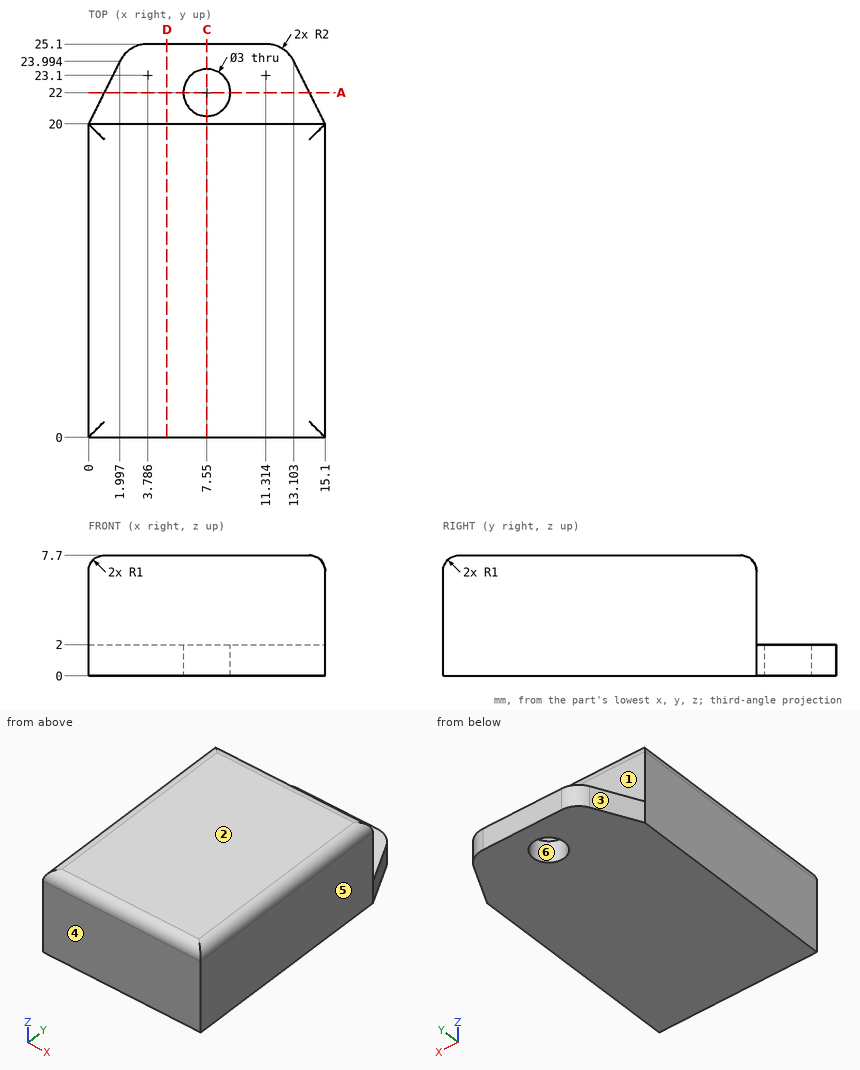
Drawing for the job (mm, zero at the part's lowest x, y, z). A direction names the side the tool comes from. Round coordinates to 2 decimals unless told otherwise and drop trailing zeros. Write each loop counter-clockwise with the first axis right and the second up, starting at its lowest first coordinate (ties: lowest second). Pieces come first, ordered by that corner, then holes. Notation, with made-up numbers: (1.5, 15) - (43.5, 15) arc R20 cw to (43.5, 26) - close; hole circle Ø11 at (-13, -30.5). An arc over 180 degrees is marked (long way). Write item = value, one per line. Start each with the question number.
Q1. Mould opens along X. For the marked faces 3, 4, 5 and 6 say: pulls with the +X half, pulls with the -X half, needs draft (parallel to the pull), parting line crosses it, or undercut.
Q2. Drop flat-ended pins along their axis: pin 1 (3 mm diameter, centred on x = 8.5, y = 5, fed in from -Z); pin 2 (2.5 mm diameter, centred on x = 6.5, y = 22, fed in from +Z). Give the stop position or say it passes through.
Q3. Band-saw the part on C-C (x = 7.55). Give the cut face in (y, z).
Q4. Band-saw the part on A-A (y = 22). Give the cut face in (x, z), then the cut area to 3 significant figures.
Q5. Which spindle directions (+Z, -Z, +X, -X, +Y, -Y) get a long thin tool onto all of the face, cutting with end or side? Do the marked faces 1 and 2. Say none if no direction does.
Q6. Probe L1, parallel to Y at x = 7.55, z = 0.85; L2, parallel to Y at x = 6.5, z = 2.25; L3, parallel to Z at x = 13.5, y = 21.25. List the from-to ranges inside material, lowest first. Write a range as from..to.
Q7. Band-saw the part on D-D (x = 5). Give the cut face in (y, z), then the cut area to 3 significant figures.
Answers below:
q1.face_3 = pulls with the -X half
q1.face_4 = needs draft
q1.face_5 = pulls with the +X half
q1.face_6 = undercut
q2.pin_1 = 0
q2.pin_2 = 2
q3.outline = (0, 0) - (20.5, 0) - (20.5, 2) - (20, 2) - (20, 6.7) arc R1 ccw to (19, 7.7) - (1, 7.7) arc R1 ccw to (0, 6.7) - close; (23.5, 0) - (25.1, 0) - (25.1, 2) - (23.5, 2) - close
q4.outline = (1, 0) - (6.05, 0) - (6.05, 2) - (1, 2) - close; (9.05, 0) - (14.1, 0) - (14.1, 2) - (9.05, 2) - close
q4.area = 20.2 mm2
q5.face_1 = +Z, +X, -X, +Y
q5.face_2 = +Z, +X, -X, +Y, -Y
q6.L1 = 0..20.5, 23.5..25.1
q6.L2 = 0..20
q6.L3 = 0..2
q7.outline = (0, 0) - (25.1, 0) - (25.1, 2) - (20, 2) - (20, 6.7) arc R1 ccw to (19, 7.7) - (1, 7.7) arc R1 ccw to (0, 6.7) - close
q7.area = 164 mm2
